Verification items for this drawing (mm, ordinates from the low corner). A direction names the side the tool comes from. Round coordinates to 2 decimals unless told otherwise and drop trailing zeros. Write each loop counter-clockwise with the first axis right and the second up, starting at its lowest first coordinate (ties: lowest second). Pieces come first, ordered by that corner, then holes. Notation, with made-up numbers: M 6.5,13 L 35.5,13 A14 ccw 35.5,30 Z; hole C 80,89 d4. An arc over 180 degrees is marked long. Write each question's results on one line, items separated by ' | '.
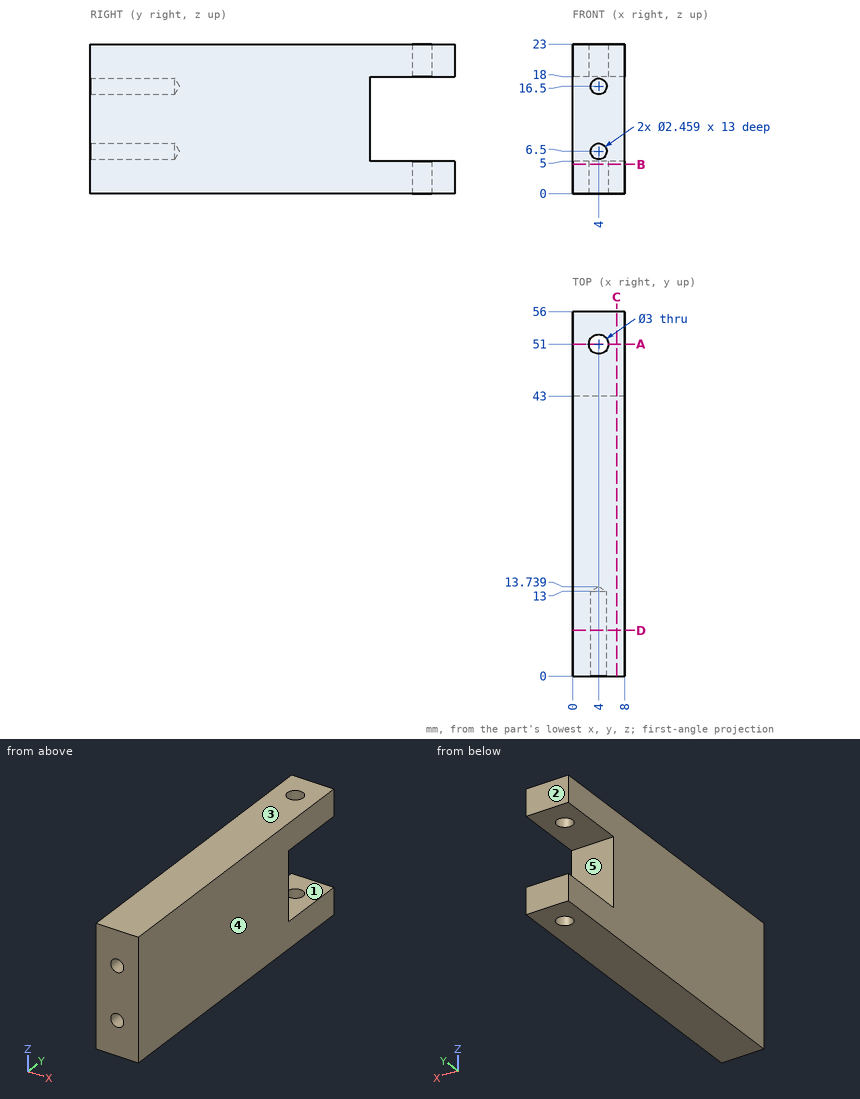
1) Depth check by flat-ended pin: P1, Ø3, axis at x = 4, z = 16.5, coming from the -Y side; P2, Ø1.5, axis at x = 4, z = 6.5, coming from the -Y side; P3, Ø3, axis at x = 6, z = 7, coming from the +Y side. Enter the tip coordinate at first touch or a pass-through.
Calculated:
P1: stops at y = 0 | P2: stops at y = 13.29 | P3: stops at y = 43
2) Access from +Z, -Z, +X, -X, +Y, -Y to the whole of each face (thin tool, end or side, straight path). Record for the marked faces 1 and 2.
Calculated:
face 1: +X, -X, +Y | face 2: +Z, -Z, +X, -X, +Y
3) Sectioned sample at D-D, the plane y = 7. Record the cut outline in (x, z).
Calculated:
outline: M 0,0 L 8,0 L 8,23 L 0,23 Z; hole C 4,6.5 d2.46; hole C 4,16.5 d2.46
4) Sectioned sample at B-B, the plane z = 4.5. Record the cut outline in (x, y), and give its area (3 significant figures).
Calculated:
outline: M 0,0 L 8,0 L 8,56 L 0,56 Z; hole C 4,51 d3 | area: 441 mm²
5) Sectioned sample at A-A, the plane y = 51. Record the cut outline in (x, z), and give its area (3 significant figures).
Calculated:
outline: M 0,0 L 2.5,0 L 2.5,5 L 0,5 Z; M 0,18 L 2.5,18 L 2.5,23 L 0,23 Z; M 5.5,0 L 8,0 L 8,5 L 5.5,5 Z; M 5.5,18 L 8,18 L 8,23 L 5.5,23 Z | area: 50.0 mm²
6) Sectioned sample at C-C, the plane x = 6.75. Record the cut outline in (y, z).
Calculated:
outline: M 0,0 L 56,0 L 56,5 L 43,5 L 43,18 L 56,18 L 56,23 L 0,23 Z
7) Draft check along Z on the marked faces 3, 4 and 5. Enter one of: pulls with the +Z half, pulls with the -Z half, needs draft (parallel to the pull), parting line crosses it, or undercut.
Calculated:
face 3: pulls with the +Z half | face 4: needs draft | face 5: undercut
8) Material ranges on line 1 (Z direction, x = 4, y = 3.5); line 2 (X direction, y = 10, z = 6.5); line 3 (Z direction, x = 7, y = 48), recorded low to high. Write a range as [from, to].
Calculated:
line 1: z = [0, 5.27], [7.73, 15.27], [17.73, 23] | line 2: x = [0, 2.77], [5.23, 8] | line 3: z = [0, 5], [18, 23]
